Input: dimensioned drawing with shaded views. Units: mm. Origin: part minimum x, y, z. Round coordinates to 2 decimals unless told otherwise and drop trailing zeros. Order: outer loops, then holes, each group sorted by start corner. A loop starts at its lowest first (then second) coordinate and runs counter-clockwise, first axis right, second up.
Item 1: Cut plane A-A on y = 25. Output: boundary loops of the cut face in (x, z).
Item 2: Cut plane B-B on x = 46.5. Output: boundary loops of the cut face in (y, z), then the cut area to 3 significant figures.
Item 3: First-contact query: pin 1 (4 mm diameter, centred on x = 3.5, y = 3.5, fed in from +Z); pin 2 (2 mm diameter, centred on y = 21, z = 2, fed in from +X). Flat tips, straight axial feed; report the tip coordinate or a pass-through.
Item 4: Cut plane D-D on x = 36. Output: boundary loops of the cut face in (y, z).
Item 5: Cut plane C-C on z = 0.65. Output: boundary loops of the cut face in (x, y), then the cut area to 3 significant figures.
Item 6: Line query: L1, parallel to Y at x = 46.5, z = 1.45; L2, parallel to Y at x = 25, z = 1.15; L3, parallel to X at y = 4, z = 1.5. Output: solid intervals per line, ascending.
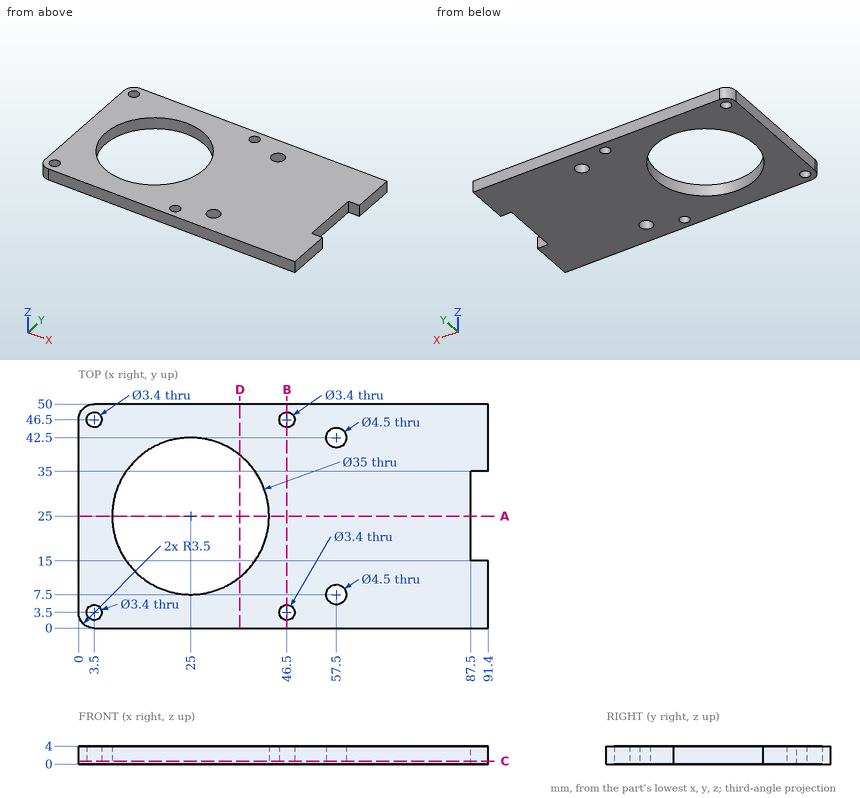
From the geometry:
1. outline: (0, 0) - (7.5, 0) - (7.5, 4) - (0, 4) - close; (42.5, 0) - (87.5, 0) - (87.5, 4) - (42.5, 4) - close
2. outline: (0, 0) - (1.8, 0) - (1.8, 4) - (0, 4) - close; (5.2, 0) - (44.8, 0) - (44.8, 4) - (5.2, 4) - close; (48.2, 0) - (50, 0) - (50, 4) - (48.2, 4) - close
2. area: 173 mm2
3. pin 1: stops at z = 4
3. pin 2: stops at x = 87.5
4. outline: (0, 0) - (11.39, 0) - (11.39, 4) - (0, 4) - close; (38.61, 0) - (50, 0) - (50, 4) - (38.61, 4) - close
5. outline: (0, 3.5) arc R3.5 ccw to (3.5, 0) - (91.4, 0) - (91.4, 15) - (87.5, 15) - (87.5, 35) - (91.4, 35) - (91.4, 50) - (3.5, 50) arc R3.5 ccw to (0, 46.5) - close; hole circle Ø3.4 at (3.5, 3.5); hole circle Ø3.4 at (3.5, 46.5); hole circle Ø35 at (25, 25); hole circle Ø3.4 at (46.5, 3.5); hole circle Ø3.4 at (46.5, 46.5); hole circle Ø4.5 at (57.5, 7.5); hole circle Ø4.5 at (57.5, 42.5)
5. area: 3,460 mm2
6. L1: y = 0 to 1.8, 5.2 to 44.8, 48.2 to 50
6. L2: y = 0 to 7.5, 42.5 to 50
6. L3: x = 0 to 1.88, 5.12 to 44.88, 48.12 to 91.4
